Build history of the part. All positions in model axes, mm. Give positions to 0.01 mm unless a question says otherwise; leave off trailing zeros. Loops run counter-clockwise (first coordinate to the right, second up) from the corner with the lowest first, then second, coordinate; pieces in that order, holes last.
1) Band-saw the part on A-A on y = -50. List the corners of the cut face in (x, z), then the cut area to 3 significant figures.
2) Band-saw the part on C-C on x = 0. List the corners of the cut face in (y, z).
3) Band-saw the part on B-B on y = -16. List the corners of the cut face in (x, z), then the cut area to 3 significant figures.
4) Wall check: line 1 (X direction, y = -30, z = 0.85); line 2 (X direction, y = -54, z = 1.15); line 3 (Y direction, x = -68, z = 0.8). Give the ranges that are in metal, low to high.
5) Two-plate mould, pull along Y, no slides. Class faces 1 (the flat face through (-1.1, -12.3, 0)), 2 (the cylindrical face through (77, 57, 1)), 3 (the cylindrical face through (70.9, -5.87, 0.99)), 4 (the cylindrical face through (70.9, -54.47, 0.99)): +Y half, -Y half, draft (parallel to the pull), parting line (faces both ways), or undercut.
6) Band-saw the part on D-D on y = 0. List the corners of the cut face in (x, z), then the cut area to 3 significant figures.
7) Flat gauge pin, fed straight in: P1, Ø2.5, axis at x = 25, y = 50, coming from the +Z side. Where does the tip first touch, or does it go through?
Autodesk Inventor part; units mm, degrees
ref_plane "YZ Plane" through (0, 0, 0) normal (1, 0, 0) x (0, 1, 0)
ref_plane "XZ Plane" through (0, 0, 0) normal (0, 1, 0) x (-1, 0, 0)
ref_plane "XY Plane" through (0, 0, 0) normal (0, 0, 1) x (1, 0, 0)
sketch "スケッチ1" plane through (0, 0, 0) normal (0, 0, 1) x (1, 0, 0)
  line L0 (-78, -59) -> (78, -59)
  line L1 (78, -59) -> (78, 59)
  line L2 (78, 59) -> (-78, 59)
  line L3 (-78, 59) -> (-78, -59)
  line L4 (-78, -59) -> (78, 59) construction
  line L5 (78, -59) -> (-78, 59) construction
  point P0 (0, 0)
  dimension "d0" = 156
  dimension "d1" = 118
extrude "プレート1" add sketch "スケッチ1" along normal blind 2
sketch "スケッチ2" plane through (0, 0, 2) normal (0, 0, 1) x (1, 0, 0)
  line L0 (-25, 30) -> (25, 30)
  line L1 (25, 30) -> (25, 50)
  line L2 (25, 50) -> (-25, 50)
  line L3 (-25, 50) -> (-25, 30)
  line L4 (-25, 30) -> (25, 50) construction
  line L5 (25, 30) -> (-25, 50) construction
  line L6 (-78, 59) -> (78, 59)
  point P0 (0, 0)
  point P1 (0, 40)
  point P2 (0, 40)
  point P3 (0, 40)
  dimension "d3" = 50
  dimension "d4" = 20
  dimension "d60" = 40
hole "穴1" at (-25, 50, 2) at (-25, 30, 2) at (25, 30, 2) at (25, 50, 2) direction (0, 0, -1) diameter 4.3 depth 2
sketch "スケッチ3" plane through (0, 0, 2) normal (0, 0, 1) x (1, 0, 0)
  line L0 (-63, 5.4) -> (-73, 5.4)
  line L1 (-73, 5.4) -> (-73, 54)
  line L2 (-73, 54) -> (-63, 54)
  line L3 (-63, 54) -> (-63, 5.4)
  line L4 (-63, 5.4) -> (-73, 54) construction
  line L5 (-73, 5.4) -> (-63, 54) construction
  line L6 (-78, 59) -> (78, 59)
  line L7 (-78, -59) -> (-78, 59)
  circle A0 centre (-68, 40) radius 6
  point P0 (0, 0)
  point P1 (-68, 29.7)
  point P2 (-68, 29.7)
  dimension "d18" = 10
  dimension "d19" = 48.6
  dimension "d20" = 14
  dimension "d31" = 19
  dimension "d47" = 68
  dimension "d48" = 12
extrude "押し出し2" cut sketch "スケッチ3" against normal blind 10 contours A0 L1 L3 | L3 A0 | A0 L1
hole "穴2" at (-63, 5.4, 2) at (-73, 5.4, 2) at (-73, 54, 2) at (-63, 54, 2) direction (0, 0, -1) diameter 4.3 depth 2
sketch "スケッチ4" plane through (0, 0, 2) normal (0, 0, 1) x (1, 0, 0)
  circle A0 centre (0, 0) radius 16
  point P0 (0, 16)
  point P1 (-13.8564, 8)
  point P2 (-13.8564, -8)
  point P3 (0, -16)
  point P4 (13.8564, -8)
  point P5 (13.8564, 8)
  dimension "d32" = 32
  dimension "d35" = 360
hole "穴3" at (0, 16, 2) at (-13.8564, 8, 2) at (-13.8564, -8, 2) at (0, -16, 2) at (13.8564, -8, 2) at (13.8564, 8, 2) direction (0, 0, -1) diameter 3.2 end through all
sketch "スケッチ5" plane through (0, 0, 2) normal (0, 0, 1) x (1, 0, 0)
  circle A0 centre (0, 0) radius 12
  dimension "d44" = 24
extrude "押し出し1" cut sketch "スケッチ5" against normal blind 10
sketch "スケッチ6" plane through (0, 0, 2) normal (0, 0, 1) x (1, 0, 0)
  point P0 (0, 0)
sketch "スケッチ7" plane through (0, 0, 2) normal (0, 0, 1) x (1, 0, 0)
  line L0 (68, 40) -> (73, 40) construction
  line L1 (68, 37.85) -> (73, 37.85)
  line L2 (73, 42.15) -> (68, 42.15)
  arc A0 (68, 42.15) -> (68, 37.85) centre (68, 40) ccw
  arc A1 (73, 37.85) -> (73, 42.15) centre (73, 40) ccw
  circle A2 centre (-68, 40) radius 6
  point P0 (0, 0)
  point P1 (70.5, 40)
  dimension "d54" = 2.15
  dimension "d55" = 5
  dimension "d57" = 68
extrude "押し出し3" cut sketch "スケッチ7" against normal blind 10 contours A0 L2 A1 L1
sketch "スケッチ8" plane through (0, 0, 0) normal (0, 0, -1) x (-1, 0, 0)
  point P0 (0, 0)
fillet "コーナーR1" radius 5 4 edges at (-78, 59, 1) (78, 59, 1) (78, -59, 1) (-78, -59, 1)
pattern_circular "円形状パターン1" count 2 over 360 about axis through (0, 0, -10) along (0, 0, 1) of "穴1", "押し出し2", "穴2", "押し出し3"
equation "\"d14\" = Thickness"
equation "\"d28\" = Thickness"
equation "\"d42\" = Thickness"
equation "\"d2\" = Thickness"
equation "\"BendRadius\" = Thickness"
equation "\"BendReliefWidth\" = Thickness"
equation "\"BendReliefDepth\" = 0.5 * Thickness"
equation "\"CornerReliefSize\" = 4 * Thickness"
equation "\"MinimumRemnant\" = 2 * Thickness"
equation "\"TransitionRadius\" = BendRadius"
equation "\"JacobiRadiusSize\" = BendRadius"
equation "\"GapSize\" = Thickness"
properties part number "carbon_plate14" material "CFRP"
Findings below:
1. outline: (-78, 0) - (-27.15, 0) - (-27.15, 2) - (-78, 2) - close; (-22.85, 0) - (22.85, 0) - (22.85, 2) - (-22.85, 2) - close; (27.15, 0) - (78, 0) - (78, 2) - (27.15, 2) - close
1. area: 295 mm2
2. outline: (-59, 0) - (-17.6, 0) - (-17.6, 2) - (-59, 2) - close; (-14.4, 0) - (-12, 0) - (-12, 2) - (-14.4, 2) - close; (12, 0) - (14.4, 0) - (14.4, 2) - (12, 2) - close; (17.6, 0) - (59, 0) - (59, 2) - (17.6, 2) - close
3. outline: (-78, 0) - (-1.6, 0) - (-1.6, 2) - (-78, 2) - close; (1.6, 0) - (78, 0) - (78, 2) - (1.6, 2) - close
3. area: 306 mm2
4. line 1: x = -78 to -27.15, -22.85 to 22.85, 27.15 to 78
4. line 2: x = -78 to 60.85, 65.15 to 70.85, 75.15 to 78
4. line 3: y = -59 to -42.15, -37.85 to 34, 46 to 59
5. face 1: draft
5. face 2: +Y half
5. face 3: undercut
5. face 4: undercut
6. outline: (-78, 0) - (-12, 0) - (-12, 2) - (-78, 2) - close; (12, 0) - (78, 0) - (78, 2) - (12, 2) - close
6. area: 264 mm2
7. P1: passes through
